Autodesk Inventor part; units mm, degrees
ref_plane "YZ Plane" through (0, 0, 0) normal (1, 0, 0) x (0, 1, 0)
ref_plane "XZ Plane" through (0, 0, 0) normal (0, 1, 0) x (-1, 0, 0)
ref_plane "XY Plane" through (0, 0, 0) normal (0, 0, 1) x (1, 0, 0)
sketch "Sketch1" plane through (0, 0, 0) normal (0, 0, 1) x (1, 0, 0)
  line L0 (-22, 22) -> (22, 22) construction
  line L1 (22, 22) -> (22, 2) construction
  line L2 (22, 2) -> (-22, 2) construction
  line L3 (-22, 2) -> (-22, 22) construction
  line L4 (-22, 22) -> (22, 2) construction
  line L5 (22, 22) -> (-22, 2) construction
  line L6 (23, 24) -> (-23, 24)
  line L7 (-23, 24) -> (-23, 0)
  line L8 (-23, 0) -> (23, 0)
  line L9 (23, 0) -> (23, 24)
  point P0 (0, 12)
  point P1 (0, 12)
  point P2 (0, 0)
  point P3 (0, 12)
  dimension "d0" = 20
  dimension "d1" = 44
  dimension "d2" = 2
  dimension "d60" = 2
  dimension "d61" = 1
  dimension "d62" = 1
extrude "Extrusion1" add sketch "Sketch1" against normal blind 3
sketch "Sketch2" plane through (-23, 0, 0) normal (0, -1, 0) x (1, 0, 0)
  line L0 (0, 0) -> (46, 0)
  line L1 (46, 0) -> (46, -16)
  line L2 (46, -16) -> (0, -16)
  line L3 (0, -16) -> (0, 0)
  line L4 (46, 0) -> (0, 0)
  line L5 (46, 0) -> (46, -3)
  line L6 (0, 0) -> (0, -3)
  point P0 (23, 0)
  dimension "d54" = 46
  dimension "d55" = 16
  dimension "d59" = 46
extrude "Extrusion2" add sketch "Sketch2" along normal blind 3
sketch "Sketch3" plane through (0, 0, 0) normal (0, 0, 1) x (1, 0, 0)
  line L0 (-21.5, 21.5) -> (21.5, 21.5) construction
  line L1 (21.5, 21.5) -> (21.5, 2.5) construction
  line L2 (21.5, 2.5) -> (-21.5, 2.5) construction
  line L3 (-21.5, 2.5) -> (-21.5, 21.5) construction
  circle A0 centre (-20.5, 20.5) radius 1 construction
  circle A1 centre (-20.5, 3.5) radius 1 construction
  circle A2 centre (20.5, 20.5) radius 1 construction
  circle A3 centre (20.5, 3.5) radius 1 construction
  line L4 (23, 24) -> (23, 0)
  line L5 (22, 22) -> (-22, 22)
  line L6 (-22, 22) -> (-22, 2)
  line L7 (-22, 2) -> (22, 2)
  line L8 (22, 2) -> (22, 22)
  point P0 (0, 0)
  point P1 (0, 2.5)
  point P2 (21.5, 12)
  point P3 (23, 12)
  point P4 (23, 0)
  point P5 (24, 3)
  dimension "d8" = 2
  dimension "d9" = 2
  dimension "d10" = 2
  dimension "d11" = 2
  dimension "d43" = 0.5
  dimension "d44" = 44
  dimension "d45" = 20
hole "Hole1" at (-20.5, 20.5, 0) at (20.5, 20.5, 0) at (20.5, 3.5, 0) at (-20.5, 3.5, 0) direction (0, 0, -1) diameter 2.4 depth 6
sketch "Sketch5" plane through (-23, 0, 0) normal (0, 1, 0) x (1, 0, 0)
  line L0 (0, 3) -> (46, 3)
  line L1 (46, 0) -> (0, 0)
  line L2 (46, 16) -> (46, 3)
  line L3 (0, 3) -> (0, 16)
  line L4 (0, 16) -> (46, 16)
  line L5 (46, 16) -> (46, 3)
  line L6 (0, 3) -> (46, 3)
  line L7 (0, 3) -> (0, 16)
  line L8 (0, 16) -> (46, 16)
  line L9 (46, 0) -> (0, 0)
  line L10 (8, 9.5) -> (38, 9.5)
  line L11 (0, 0) -> (0, 3)
  line L12 (46, 3) -> (46, 0)
  line L13 (0, 0) -> (0, 3)
  line L14 (46, 3) -> (46, 0)
  point P0 (23, 9.5)
  point P1 (23, 16)
  dimension "d56" = 13
  dimension "d57" = 6.5
  dimension "d58" = 30
hole "Hole2" at (-15, 0, -9.5) at (15, 0, -9.5) direction (0, -1, 0) diameter 3.4 depth 6
chamfer "Chamfer2" distance 3 angle 45 4 edges at (-23, 24, -1.5) (23, 24, -1.5) (23, -1.5, -16) (-23, -1.5, -16)
sketch "Sketch6" plane through (0, 0, 0) normal (0, 0, 1) x (1, 0, 0)
  circle A0 centre (-20.5, 20.5) radius 1.2
  circle A1 centre (-20.5, 20.5) radius 2
  circle A2 centre (20.5, 20.5) radius 1.2
  circle A3 centre (20.5, 20.5) radius 2
  circle A4 centre (20.5, 3.5) radius 1.2
  circle A5 centre (20.5, 3.5) radius 2
  circle A6 centre (-20.5, 3.5) radius 1.2
  circle A7 centre (-20.5, 3.5) radius 2
  point P0 (0, 0)
  dimension "d46" = 4
  dimension "d47" = 4
  dimension "d49" = 4
  dimension "d50" = 4
extrude "Extrusion3" add sketch "Sketch6" along normal blind 7
equation "\"d60\" = d2"
equation "\"d62\" = d61"
equation "\"d54\" = d59"
equation "\"d44\" = d1"
equation "\"d45\" = d0"
equation "\"d57\" = 0.5 * d56"
equation "\"d46\" = d50"
equation "\"d47\" = d50"
equation "\"d49\" = d50"
properties part number "ultrasonic mount (front) v2"
Geometry: final body of the model. Coordinates: model frame, mm. A direction names the side the tool comes from. Round coordinates to 2 decimals unless told otherwise and drop trailing zeros. Loops run counter-clockwise (first coordinate to the right, second up) from the corner with the lowest first, then second, coordinate; pieces in that order, holes last.
Q1. Section D-D on y = 14.25. Return loops of the section in (x, z), plus the area to 3 significant figures.
Q2. Pull-direction query (Y, two-part tool) for faces 4 (the flat face through (0, 24, -1)), 5 (the flat face through (23, 6.3, -2.6)), 6 (the cylindrical face through (20.24, 18.517, 3.451)); classes: released by +Y, released by -Y, zero draft, split by the parting line, or undercut.
Q3. Material intervals for L1, parallel to Y at x = 20.5, z = 1.5; L2, parallel to Z at x = -15, y = -1.9; L3, parallel to Y at x = 20.5, z = -1, sorted ascending.
Q4. Pin query (flat end, axial travel): P1, Ø4, axis at x = -12.5, z = -9, coming from the +Y side; P2, Ø8, axis at x = -2.5, y = 5.5, coming from the -Z side; P3, Ø2, axis at x = 20.5, y = 3.5, coming from the +Z side; P4, Ø2, axis at x = 13.5, y = 18, coming from the +Z side. Return the tip coordinate at first contact, or that it passes through.
Q5. Access query for faces 1 (the cylindrical face through (18.9, 4.7, 3.5)), 2 (the flat face through (0, 12, -3)), 3 (the cylindrical face through (-19.934, 2.442, 1.93)). Directions: +Z, -Z, +X, -X, +Y, -Y. A direction counts if a zero-diameter tool reaches every point of the face in a straight line with its end or side. Return the directions, or none.
Q6. Section B-B on x = -15. Return loops of the section in (y, z).
Q7. Section C-C on z = -9.5. Return loops of the section in (x, y), plus the area to 3 significant figures.
Q8. Section A-A on z = 4.25. Return loops of the section in (x, y), plus the area to 3 significant figures.
Evaluation:
1. outline: (-23, -3) - (23, -3) - (23, 0) - (-23, 0) - close
1. area: 138 mm2
2. face 4: released by +Y
2. face 5: zero draft
2. face 6: undercut
3. L1: y = 1.5 to 2.3, 4.7 to 5.5, 18.5 to 19.3, 21.7 to 22.5
3. L2: z = -16 to -11.2, -7.8 to 0
3. L3: y = -3 to 2.3, 4.7 to 19.3, 21.7 to 23.5
4. P1: stops at y = 0
4. P2: stops at z = -3
4. P3: passes through
4. P4: stops at z = 0
5. face 1: +Z
5. face 2: -Z, +X, -X, +Y
5. face 3: +Z, -Z
6. outline: (-3, -16) - (0, -16) - (0, -11.2) - (-3, -11.2) - close; (-3, -7.8) - (0, -7.8) - (0, -3) - (24, -3) - (24, 0) - (-3, 0) - close
7. outline: (-23, -3) - (-16.7, -3) - (-16.7, 0) - (-23, 0) - close; (-13.3, -3) - (13.3, -3) - (13.3, 0) - (-13.3, 0) - close; (16.7, -3) - (23, -3) - (23, 0) - (16.7, 0) - close
7. area: 118 mm2
8. outline: circle Ø4 at (-20.5, 3.5); circle Ø4 at (-20.5, 20.5); circle Ø4 at (20.5, 3.5); circle Ø4 at (20.5, 20.5); hole circle Ø2.4 at (-20.5, 3.5); hole circle Ø2.4 at (-20.5, 20.5); hole circle Ø2.4 at (20.5, 3.5); hole circle Ø2.4 at (20.5, 20.5)
8. area: 32.2 mm2
